Geometry check sheet. Reference: the model listing, model coordinates, mm. Round coordinates to 2 decimals unless told otherwise and drop trailing zeros. Loops run counter-clockwise (first coordinate to the right, second up) from the corner with the lowest first, then second, coordinate; pieces in that order, holes last. Notation, with made-up numbers: (45, 70.25) -> (89, 70.25) arc R7 cw to (89, 74.25) -> close; hole circle Ø1 at (83.25, 40.25). An arc over 180 degrees is marked (long way). Use one line per item in the form item = value.
from build123d import *

# Parameters (mm, degrees)
F0_W     = 31.75
F0_H     = 31.75
F1_DEPTH = 3.175
F3_D     = 0.79375
F5_D     = 1.5875


# Not quite as in the source:
# - a feature names something its author has since deleted; it is built from what else it names


with BuildPart() as f1:
    # F0 (on Front) → F1 (new body, symmetric)
    with BuildSketch(Plane.XZ):
        Rectangle(F0_W, F0_H)
    extrude(amount=F1_DEPTH, both=True)

    # F3 (through all)
    with Locations(Plane.XZ.offset(3.175)):
        with Locations((0, 0), (0, 2.38125), (2.0622229928, 1.190625), (2.0622229928, -1.190625), (0, -2.38125), (-2.0622229928, -1.190625), (-2.0622229928, 1.190625), (-4.8118536498, 2.778125), (-2.778125, 4.8118536498), (0, 5.55625), (2.778125, 4.8118536498), (4.8118536498, 2.778125), (5.55625, 0), (4.8118536498, -2.778125), (2.778125, -4.8118536498), (0, -5.55625), (-2.778125, -4.8118536498), (-4.8118536498, -2.778125), (-5.55625, 0)):
            Hole(F3_D / 2)

    # F5 (through all)
    with Locations(Plane.XZ.offset(3.175)):
        with Locations((-13.335, 13.335), (-13.335, -13.335), (13.335, 13.335), (13.335, -13.335)):
            Hole(F5_D / 2)


solid = f1.part
1. Material ranges on line 1 along Z through (x, y) = (2, -1) (3 decimals); line 2 along X through (y, z) = (1.75, -5) (3 decimals); line 3 along Z through (x, y) = (-5.5, -3) (3 decimals), recorded low to high.
Return value:
line_1 = -15.875 to -1.583, -0.799 to 0.799, 1.583 to 15.875
line_2 = -15.875 to -3.128, -2.429 to 2.429, 3.128 to 15.875
line_3 = -15.875 to -0.393, 0.393 to 15.875
2. Section check C-C (y = -1.25). Count the separate pieces of the cut face and the enclosed holes in it, then the cut area to 3 significant figures.
Return value:
separate_pieces = 1
enclosed_holes = 23
area = 991 mm2
3. Section check B-B (z = 0). Record the boundary of the cut face in (x, y) (3 decimals), then the cut area to 3 significant figures.
Return value:
outline = (-15.875, -3.175) -> (-5.953, -3.175) -> (-5.953, 3.175) -> (-15.875, 3.175) -> close; (-5.159, -3.175) -> (-0.397, -3.175) -> (-0.397, 3.175) -> (-5.159, 3.175) -> close; (0.397, -3.175) -> (5.159, -3.175) -> (5.159, 3.175) -> (0.397, 3.175) -> close; (5.953, -3.175) -> (15.875, -3.175) -> (15.875, 3.175) -> (5.953, 3.175) -> close
area = 186 mm2
4. Section check A-A (x = 0). Record the boundary of the cut face in (y, z) (3 decimals).
Return value:
outline = (-3.175, -15.875) -> (3.175, -15.875) -> (3.175, -5.953) -> (-3.175, -5.953) -> close; (-3.175, -5.159) -> (3.175, -5.159) -> (3.175, -2.778) -> (-3.175, -2.778) -> close; (-3.175, -1.984) -> (3.175, -1.984) -> (3.175, -0.397) -> (-3.175, -0.397) -> close; (-3.175, 0.397) -> (3.175, 0.397) -> (3.175, 1.984) -> (-3.175, 1.984) -> close; (-3.175, 2.778) -> (3.175, 2.778) -> (3.175, 5.159) -> (-3.175, 5.159) -> close; (-3.175, 5.953) -> (3.175, 5.953) -> (3.175, 15.875) -> (-3.175, 15.875) -> close
5. Mould release check, pull along X, two halves, no side actions. Record for faces 1 (the flat face through (-15.875, 0, 0)), 2 (the cylindrical face through (13.965, 0.044, -13.818)), 3 (the flat face through (0, 0, 15.875)): released by +X, released by -X, zero draft, split by the parting line, or undercut.
Return value:
face_1 = released by -X
face_2 = undercut
face_3 = zero draft
